Here's how the part is built. I have some questions about the finished solid (model axes, mm). Face numbers are marked on the shaded views. A direction names the side the tool comes from. Round coordinates to 2 decimals unless told otherwise and drop trailing zeros. Write each loop counter-clockwise with the first axis right and the second up, starting at its lowest first coordinate (ties: lowest second). Pieces come first, ordered by that corner, then holes. Notation, with made-up numbers: (-30, -6) - (-20, -6) arc R17 cw to (-20, 24) - close; hole circle Ø6 at (46, 89). An arc over 180 degrees is marked (long way). Write item = value, one per line. Start each with the question number.
Item 1: If we section it at C-C (z = 27): Please give me the cut outline in (x, y), and give its area (3 significant figures).
Item 2: For P1, Ø6, axis at x = 2, z = 17, coming from the +Y side; P2, Ø4, axis at y = 3, z = 28, coming from the -X side; P3, Ø4, axis at x = -7, z = 11, coming from the +Y side, each with a flat end and sliding along its axis, tell me the tip position at first contact or that it passes through.
Item 3: If we section it at B-B (y = 0): Please give me the cut outline in (x, z), and give its area (3 significant figures).
Item 4: If we section it at A-A (x = 0): Please give me the cut outline in (y, z), and give its area (3 significant figures).
Item 5: Which directions (+Z, -Z, +X, -X, +Y, -Y) give clear straight access to the entire face, cutting with the end or side of a thin tool? Please do the marked faces 1 and 2.
Item 6: If I drill on line 1 along Z through (x, y) = (-6, -10); line 2 along Y through (x, z) = (0, 0.5); line 3 along Y through (x, z) = (0, 1.3), over which ranges is the centre line in solid material (lowest first)? Write a range as [from, to].
```python
from build123d import *

# Parameters (mm, degrees)
SKETCH_R           = 20
PAD_DEPTH          = 2
SKETCH001_R        = 7.5
PAD001_DEPTH       = 38
SKETCH002_R        = 1.7
HOLE_DEPTH         = 140.565065
POLARPATTERN_COUNT = 3
FILLET_R           = 3
CHAMFER_SIZE       = 1


with BuildPart() as part:
    # Sketch → Pad (new body)
    with BuildSketch(Plane.XY):
        Circle(SKETCH_R)
    extrude(amount=PAD_DEPTH)

    # Sketch001 (on Face3 of Pad) → Pad001 (join)
    with BuildSketch(Plane.XY.offset(2)):
        Circle(SKETCH001_R)
    extrude(amount=PAD001_DEPTH)

    # Sketch002 (on Face3 of Pad001) → Hole (cut, through all)
    with BuildSketch(Plane.XY.offset(2)):
        with Locations((0, 15)):
            Circle(SKETCH002_R)
    hole = extrude(amount=-HOLE_DEPTH, mode=Mode.SUBTRACT)

    # PolarPattern: Hole ×3 about axis
    polarpattern_axis = Axis((0, 0, 2), (0, 0, 1))
    for i in range(1, POLARPATTERN_COUNT):
        add(hole.rotate(polarpattern_axis, i * 360 / POLARPATTERN_COUNT), mode=Mode.SUBTRACT)

    # Fillet
    fillet_edges = [part.edges().sort_by_distance(p)[0] for p in [
        (-7.5, 0, 2),
    ]]
    fillet(fillet_edges, radius=FILLET_R)

    # Chamfer
    chamfer_edges = [part.edges().sort_by_distance(p)[0] for p in [
        (-20, 0, 2),
    ]]
    chamfer(chamfer_edges, length=CHAMFER_SIZE)


solid = part.part
```
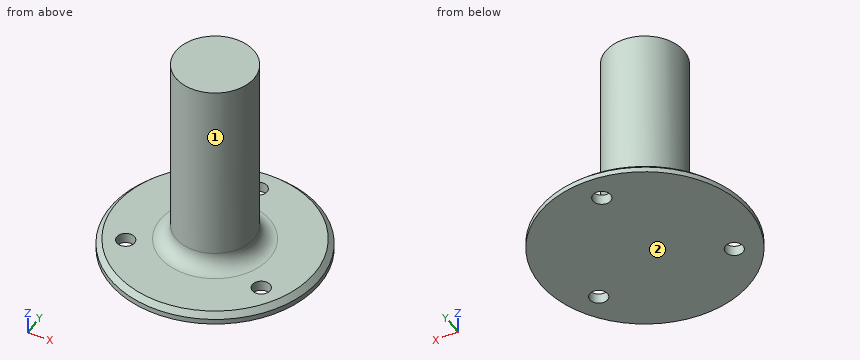
Reply:
q1.outline = circle Ø15 at (0, 0)
q1.area = 177 mm2
q2.P1 = 7.5
q2.P2 = -7.43
q2.P3 = 5.59
q3.outline = (-20, 0) - (20, 0) - (20, 1) - (19, 2) - (10.5, 2) arc R3 cw to (7.5, 5) - (7.5, 40) - (-7.5, 40) - (-7.5, 5) arc R3 cw to (-10.5, 2) - (-19, 2) - (-20, 1) - close
q3.area = 653 mm2
q4.outline = (-20, 0) - (13.3, 0) - (13.3, 2) - (10.5, 2) arc R3 cw to (7.5, 5) - (7.5, 40) - (-7.5, 40) - (-7.5, 5) arc R3 cw to (-10.5, 2) - (-19, 2) - (-20, 1) - close; (16.7, 0) - (20, 0) - (20, 1) - (19, 2) - (16.7, 2) - close
q4.area = 646 mm2
q5.face_1 = +Z
q5.face_2 = -Z, +X, -X, +Y, -Y
q6.line_1 = [0, 2]
q6.line_2 = [-20, 13.3], [16.7, 20]
q6.line_3 = [-19.7, 13.3], [16.7, 19.7]
